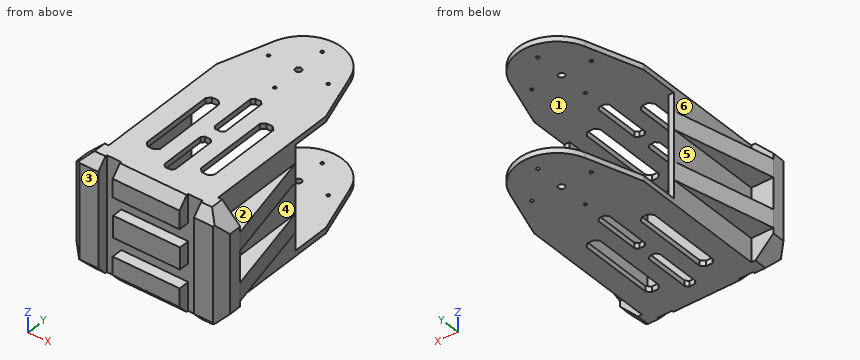
from build123d import *

# Parameters (mm, degrees)
SKETCH_1_W             = 60.6
SKETCH_1_H             = 63.3
SKETCH_1_W_2           = 54.6
SKETCH_1_H_2           = 57.3
EXTRUDE_1_DEPTH        = 60
SKETCH_2_W             = 60.6
SKETCH_2_H             = 3
EXTRUDE_2_DEPTH        = 65
CUT_EXTRUDE_1_DEPTH    = 65
SKETCH_9_R             = 1.725
CUT_EXTRUDE_4_DEPTH    = 80
SKETCH_10_W            = 85
SKETCH_10_H            = 63.3
EXTRUDE_3_DEPTH        = 6
CHAMFER_1_SIZE         = 10
CHAMFER_2_SIZE         = 5
CHAMFER_2_SIZE2        = 5.553062574
CHAMFER_2_PART_2_SIZE  = 5
CHAMFER_2_PART_2_SIZE2 = 5.553062574
CHAMFER_2_PART_3_SIZE  = 5
CHAMFER_2_PART_3_SIZE2 = 5.553062574
CHAMFER_2_PART_4_SIZE  = 5
CHAMFER_2_PART_4_SIZE2 = 5.553062574
SKETCH_12_W            = 8
SKETCH_12_H            = 6
CUT_EXTRUDE_5_DEPTH    = 80
SKETCH_13_W            = 37
SKETCH_13_H            = 10
CUT_EXTRUDE_7_DEPTH    = 6
SKETCH_14_W            = 37
SKETCH_14_H            = 12
CUT_EXTRUDE_8_DEPTH    = 0.3
EXTRUDE_4_DEPTH        = 5
MIRROR_2_COPY_1_DEPTH  = 5
SKETCH_8_R             = 0.84
CUT_EXTRUDE_9_DEPTH    = 80
CUT_EXTRUDE_10_DEPTH   = 80


with BuildPart() as part:
    # 草图1 → 凸台-拉伸1 (new body)
    with BuildSketch(Plane(origin=(0, 0, 0), x_dir=(1, 0, 0), z_dir=(0, 1, 0))):
        Rectangle(SKETCH_1_W, SKETCH_1_H)
        Rectangle(SKETCH_1_W_2, SKETCH_1_H_2, mode=Mode.SUBTRACT)
    extrude(amount=EXTRUDE_1_DEPTH)

    # 草图2 → 凸台-拉伸2 (add)
    with BuildSketch(Plane(origin=(0, 60, 0), x_dir=(1, 0, 0), z_dir=(0, 1, 0))):
        with Locations((0, 30.15)):
            Rectangle(SKETCH_2_W, SKETCH_2_H)
        with Locations((0, -30.15)):
            Rectangle(SKETCH_2_W, SKETCH_2_H)
    extrude(amount=EXTRUDE_2_DEPTH)

    # 草图3 → 切除-拉伸1 (cut)
    with BuildSketch(Plane(origin=(0, 0, -31.65), x_dir=(-1, 0, 0), z_dir=(0, 0, -1))):
        with BuildLine():
            Line((-30.3, 81), (-20.919056551, 109.811246068))
            ThreePointArc((-20.919056551, 109.811246068), (0, 125), (20.919056551, 109.811246068))
            Line((20.919056551, 109.811246068), (30.3, 81))
            Line((30.3, 81), (30.3, 183))
            Line((30.3, 183), (-30.3, 125))
            Line((-30.3, 125), (-30.3, 81))
        make_face()
    extrude(amount=-CUT_EXTRUDE_1_DEPTH, mode=Mode.SUBTRACT)

    # 草图9 → 切除-拉伸4 (cut)
    with BuildSketch(Plane(origin=(0, 0, -31.65), x_dir=(-1, 0, 0), z_dir=(0, 0, -1))):
        with Locations((0, 100)):
            Circle(SKETCH_9_R)
    extrude(amount=-CUT_EXTRUDE_4_DEPTH, mode=Mode.SUBTRACT)

    # 草图10 → 凸台-拉伸3 (add, symmetric)
    with BuildSketch(Plane.XZ):
        Rectangle(SKETCH_10_W, SKETCH_10_H)
    extrude(amount=EXTRUDE_3_DEPTH, both=True)

    # 倒角1
    chamfer_1_edges = [part.edges().sort_by_distance(p)[0] for p in [
        (42.5, 0, 31.65),
        (-42.5, 0, -31.65),
        (42.5, 0, -31.65),
        (-42.5, 0, 31.65),
    ]]
    chamfer(chamfer_1_edges, length=CHAMFER_1_SIZE)

    # 倒角2
    chamfer_2_edges = [part.edges().sort_by_distance(p)[0] for p in [
        (42.5, -6, 0),
    ]]
    chamfer_2_side = [part.faces().sort_by_distance(p)[0] for p in [
        (42.5, 0, 0),
    ]]
    chamfer(chamfer_2_edges, length=CHAMFER_2_SIZE, length2=CHAMFER_2_SIZE2, reference=chamfer_2_side[0])

    # 倒角2 part 2
    chamfer_2_part_2_edges = [part.edges().sort_by_distance(p)[0] for p in [
        (-42.5, -6, 0),
    ]]
    chamfer_2_part_2_side = [part.faces().sort_by_distance(p)[0] for p in [
        (-42.5, 0, 0),
    ]]
    chamfer(chamfer_2_part_2_edges, length=CHAMFER_2_PART_2_SIZE, length2=CHAMFER_2_PART_2_SIZE2, reference=chamfer_2_part_2_side[0])

    # 倒角2 part 3
    chamfer_2_part_3_edges = [part.edges().sort_by_distance(p)[0] for p in [
        (0, -6, -31.65),
    ]]
    chamfer_2_part_3_side = [part.faces().sort_by_distance(p)[0] for p in [
        (0, 53.785060823, -31.65),
    ]]
    chamfer(chamfer_2_part_3_edges, length=CHAMFER_2_PART_3_SIZE, length2=CHAMFER_2_PART_3_SIZE2, reference=chamfer_2_part_3_side[0])

    # 倒角2 part 4
    chamfer_2_part_4_edges = [part.edges().sort_by_distance(p)[0] for p in [
        (0, -6, 31.65),
    ]]
    chamfer_2_part_4_side = [part.faces().sort_by_distance(p)[0] for p in [
        (0, 53.785060823, 31.65),
    ]]
    chamfer(chamfer_2_part_4_edges, length=CHAMFER_2_PART_4_SIZE, length2=CHAMFER_2_PART_4_SIZE2, reference=chamfer_2_part_4_side[0])

    # 草图12 → 切除-拉伸5 (cut)
    with BuildSketch(Plane(origin=(0, 0, -31.65), x_dir=(-1, 0, 0), z_dir=(0, 0, -1))):
        with Locations((-22.5, -3)):
            Rectangle(SKETCH_12_W, SKETCH_12_H)
        with Locations((22.5, -3)):
            Rectangle(SKETCH_12_W, SKETCH_12_H)
    extrude(amount=-CUT_EXTRUDE_5_DEPTH, mode=Mode.SUBTRACT)

    # 草图13 → 切除-拉伸7 (cut)
    with BuildSketch(Plane.XZ.offset(6)):
        with Locations((0, 11)):
            Rectangle(SKETCH_13_W, SKETCH_13_H)
        with Locations((0, -11)):
            Rectangle(SKETCH_13_W, SKETCH_13_H)
    extrude(amount=-CUT_EXTRUDE_7_DEPTH, mode=Mode.SUBTRACT)

    # 草图14 → 切除-拉伸8 (cut)
    with BuildSketch(Plane.XZ.offset(6)):
        Rectangle(SKETCH_14_W, SKETCH_14_H)
    extrude(amount=-CUT_EXTRUDE_8_DEPTH, mode=Mode.SUBTRACT)

    # 草图18 → 凸台-拉伸4 (add, symmetric)
    with BuildSketch(Plane(origin=(0, 0, -13.65), x_dir=(-1, 0, 0), z_dir=(0, 0, -1))):
        Polygon((30.3, 60), (42.5, 6), (30.3, 6), align=None)
    extrude_4 = extrude(amount=EXTRUDE_4_DEPTH, both=True)

    # 镜向1: 凸台-拉伸4 across plane
    add(extrude_4.mirror(Plane.XY))

    # 镜向2: 凸台-拉伸4 across plane
    add(extrude_4.mirror(Plane(origin=(0, 0, 0), x_dir=(0, 0, 1), z_dir=(1, 0, 0))))

    # 镜向2 copy 1 sketch → 镜向2 copy 1 (add, symmetric)
    with BuildSketch(Plane.XY.offset(13.65)):
        Polygon((30.3, 60), (42.5, 6), (30.3, 6), align=None)
    extrude(amount=MIRROR_2_COPY_1_DEPTH, both=True)

    # 草图8 → 切除-拉伸9 (cut)
    with BuildSketch(Plane.XY.offset(31.65)):
        with Locations((0, 116.5)):
            Circle(SKETCH_8_R)
        with Locations((16.5, 100)):
            Circle(SKETCH_8_R)
        with Locations((0, 83.5)):
            Circle(SKETCH_8_R)
        with Locations((-16.5, 100)):
            Circle(SKETCH_8_R)
    extrude(amount=-CUT_EXTRUDE_9_DEPTH, mode=Mode.SUBTRACT)

    # 草图19 → 切除-拉伸10 (cut)
    with BuildSketch(Plane(origin=(0, 0, -31.65), x_dir=(-1, 0, 0), z_dir=(0, 0, -1))):
        Polygon((-1.5, 44), (1.5, 44), (3, 45.5), (3, 70.5), (1.5, 72), (-1.5, 72), (-3, 70.5), (-3, 45.5), align=None)
        Polygon((-16.75, 61), (-13.25, 61), (-11.25, 59), (-11.25, 18), (-13.25, 16), (-16.75, 16), (-18.75, 18), (-18.75, 59), align=None)
        Polygon((-3, 10.5), (-3, 35.5), (-1.5, 37), (1.5, 37), (3, 35.5), (3, 10.5), (1.5, 9), (-1.5, 9), align=None)
        Polygon((13.25, 16), (11.25, 18), (11.25, 59), (13.25, 61), (16.75, 61), (18.75, 59), (18.75, 18), (16.75, 16), align=None)
    extrude(amount=-CUT_EXTRUDE_10_DEPTH, mode=Mode.SUBTRACT)


solid = part.part
Read the model definition and answer for the solid it produces. Units are mm, in the model's axes. Face numbers are marked on the shaded views. A direction names the side the tool comes from. Coordinates: 2 decimals unless noted, no trailing zeros. Write each loop counter-clockwise with the first axis right and the second up, starting at its lowest first coordinate (ties: lowest second). Pieces come first, ordered by that corner, then holes. Notation, with made-up numbers: M -30,74.5 L 9,74.5 A16 ccw 9,86.5 Z; hole C 6.25,83.25 d9. An arc over 180 degrees is marked long. Use a Markdown table: item, result.
Q1. Straight lines are drawn through the part: L1, parallel to Z at x = -2.5, y = 75; L2, parallel to X at y = 39.5, z = 4; L3, parallel to Y at x = 16.5, z = -30.95. For each, find the intervals that lie inside material, in ascending order. Write a range as [from, to].
Answer block:
| item | result |
|---|---|
| L1 | z = [-31.65, -28.65], [28.65, 31.65] |
| L2 | x = [-30.3, -27.3], [27.3, 30.3] |
| L3 | y = [-1.63, 16], [61, 99.16], [100.84, 117.55] |
Q2. Which of the six approach directions +Z, -Z, +X, -X, +Y, -Y give full straight-line access (tool end or side, diameter ignored) to the marked faces 4, 5 and 6?
Answer block:
| item | result |
|---|---|
| face 4 | +X, +Y |
| face 5 | -X, +Y |
| face 6 | +Z, -X, +Y |
Q3. The part is cut by section A-A, the plane z = -1. Write down the section's boundary in (x, y), then the cut area to 3 significant figures.
Answer block:
| item | result |
|---|---|
| outline | M -42.5,-1 L -36.95,-6 L -26.5,-6 L -26.5,0 L -18.5,0 L -18.5,-5.7 L 18.5,-5.7 L 18.5,0 L 26.5,0 L 26.5,-6 L 36.95,-6 L 42.5,-1 L 42.5,6 L 30.3,6 L 30.3,60 L 27.3,60 L 27.3,6 L -27.3,6 L -27.3,60 L -30.3,60 L -30.3,6 L -42.5,6 Z |
| area | 1,210 mm2 |
Q4. The part is cut by section B-B, the plane z = 11. Write down the section's boundary in (x, y).
Answer block:
| item | result |
|---|---|
| outline | M -42.5,-1 L -36.95,-6 L -26.5,-6 L -26.5,0 L 26.5,0 L 26.5,-6 L 36.95,-6 L 42.5,-1 L 42.5,6 L 30.3,60 L 27.3,60 L 27.3,6 L -27.3,6 L -27.3,60 L -30.3,60 L -42.5,6 Z |
Q5. Determine the mould class of the marked faces 1, 2 and 3 for opening direction Z: released by +Z, released by -Z, zero draft, split by the parting line, or undercut.
Answer block:
| item | result |
|---|---|
| face 1 | undercut |
| face 2 | released by +Z |
| face 3 | zero draft |
Q6. Each of these flat-tipped pins is pushed along its axis until it touches: pin 1 Ø6 at (x, y) = (39, 43.5) entering from +Z; pin 2 Ø6 at (x, z) = (27, 6) entering from +Y; pin 3 Ø2.5 at (y, z) = (39.5, -29.5) entering from +X; pin 4 Ø3.5 at (x, z) = (0.5, 31) entering from -Y. Where does it stop, or does it pass through?
Answer block:
| item | result |
|---|---|
| pin 1 | passes through |
| pin 2 | stops at y = 60 |
| pin 3 | stops at x = 30.3 |
| pin 4 | stops at y = -3.16 |
